Input: part model. Units: mm. Frame: model coordinates. A direction names the side the tool comes from. Round coordinates to 2 decimals unless told otherwise and drop trailing zeros. Loops run counter-clockwise (first coordinate to the right, second up) from the corner with the lowest first, then second, coordinate; pieces in that order, holes last. Notation, with made-up numbers: (10, 41) -> (34, 41) arc R15 cw to (34, 69) -> close; hole circle Ø8 at (18.5, -15). An arc over 180 degrees is marked (long way). Answer as a JSON object with one key per item and string values. Group by question number.
Item 1: Set-up query: faces 1 (the flat face through (5, -2, -19.451)), 2 (the cylindrical face through (-9.76, -2.17, -18.18)), 3 (the flat face through (2.6, -7.2, -9.951)). Return all of +Z, -Z, +X, -X, +Y, -Y with unobstructed straight access to the full face (end or side cutting, diameter ignored); none if empty.
Item 2: Section query A-A on y = 0. Return loops of the section in (x, z).
Item 3: Draft query along X for faces 4 (the cylindrical face through (-4.88, -1.08, -13.29)), 5 (the cylindrical face through (0.33, -7.493, -13.402)), 6 (the flat face through (7, 4, -16.951)). Return one class per face: released by +X, released by -X, zero draft, split by the parting line, or undercut.
Item 4: Pin query (flat end, axial travel): pin 1 (12 mm diameter, centred on x = -2, y = -2, fed in from -Z); pin 2 (3 mm diameter, centred on y = 1.5, z = -17.5, fed in from -X); pin 3 (5 mm diameter, centred on y = 4, z = -14, fed in from -X); pin 4 (1.5 mm diameter, centred on y = 5.5, z = -12, fed in from -X). Return the tip coordinate at first contact, or that it passes through.
Item 5: Material intervals for line 1 (Z direction, x = -8.5, y = 2.25); line 2 (X direction, y = 0, z = -13.75); line 3 (Y direction, x = -1.5, z = -15.25), sorted ascending. Write a range as [from, to].
Item 6: Section query C-C on z = -15.25. Return loops of the section in (x, y).
from build123d import *

# Parameters (mm, degrees)
F2_SIZE = 1


with BuildPart() as f1:
    # F0 (on Right) → F1 (revolve)
    with BuildSketch(Plane.YZ):
        Polygon((5, -6.950552), (5, -19.450552), (10, -19.450552), (10, -16.950552), (7.5, -16.950552), (7.5, -9.950552), (11, -9.950552), (11, -6.950552), align=None)
    revolve(axis=Axis((0, 0, -7.205679), (0, 0, -1)))

    # F2
    f2_edges = [f1.edges().sort_by_distance(p)[0] for p in [
        (0, -11, -6.950552),
    ]]
    chamfer(f2_edges, length=F2_SIZE)


solid = f1.part
Solved:
{
 "1": {"face 1": "-Z, +X, -X, +Y, -Y", "face 2": "-Z", "face 3": "none"},
 "2": {"outline": "(-11, -9.95) -> (-7.5, -9.95) -> (-7.5, -16.95) -> (-10, -16.95) -> (-10, -19.45) -> (-5, -19.45) -> (-5, -6.95) -> (-10, -6.95) -> (-11, -7.95) -> close; (5, -19.45) -> (10, -19.45) -> (10, -16.95) -> (7.5, -16.95) -> (7.5, -9.95) -> (11, -9.95) -> (11, -7.95) -> (10, -6.95) -> (5, -6.95) -> close"},
 "3": {"face 4": "undercut", "face 5": "split by the parting line", "face 6": "zero draft"},
 "4": {"pin 1": "z = -19.45", "pin 2": "x = -10", "pin 3": "x = -7.35", "pin 4": "x = -5.8"},
 "5": {"line 1": "[-19.45, -16.95], [-9.95, -6.95]", "line 2": "[-7.5, -5], [5, 7.5]", "line 3": "[-7.35, -4.77], [4.77, 7.35]"},
 "6": {"outline": "circle Ø15 at (0, 0); hole circle Ø10 at (0, 0)"}
}
